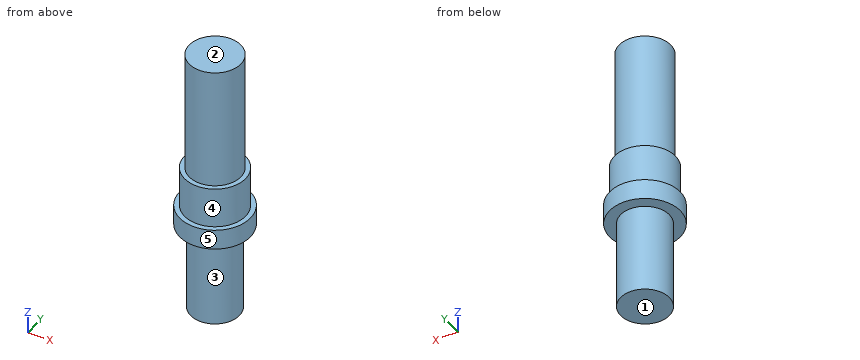
from build123d import *

# Parameters (mm, degrees)
SKETCH5_R             = 6.35
OUTSIDE_EXTRUDE_DEPTH = 30
INSIDE_START          = 2
SKETCH6_R             = 6
INSIDE_EXTRUDE_DEPTH  = 2


with BuildPart() as part:
    # Sketch3 → Initial Resolve -- Exact Length (revolve)
    with BuildSketch(Plane(origin=(0, 0, 0), x_dir=(0, 0, -1), z_dir=(1, 0, 0))):
        Polygon((9.998219577, 8.7), (14.998219577, 8.7), (14.998219577, 6), (34.998219577, 6), (34.998219577, 0), (0, 0), (-0.001780423, 0), (-0.001780423, 7.5), (9.998219577, 7.5), align=None)
    revolve(axis=Axis((0, 0, -34.998219577), (0, 0, 1)))

    # Sketch5 → Outside Extrude (add)
    with BuildSketch(Plane.XY.offset(0.001780423)):
        Circle(SKETCH5_R)
    extrude(amount=OUTSIDE_EXTRUDE_DEPTH)

    # Sketch6 → Inside Extrude (add)
    with BuildSketch(Plane(origin=(0, 0, -34.998219577), x_dir=(-1, 0, 0), z_dir=(0, 0, -1)).offset(INSIDE_START)):
        with Locations(Location((0, 0, 0), (0, 0, 90))):
            Circle(SKETCH6_R)
    extrude(amount=-INSIDE_EXTRUDE_DEPTH)


solid = part.part
Model file for the job. Use its own axes, mm. Face numbers are marked on the shaded views. A direction names the side the tool comes from. Give positions to 0.01 mm unless a question says otherwise; leave off trailing zeros. Loops run counter-clockwise (first coordinate to the right, second up) from the corner with the lowest first, then second, coordinate; pieces in that order, holes last.
1) Wall check: line 1 (Z direction, x = 4.5, y = 5.75); line 2 (Y direction, x = -5.25, z = 2); line 3 (X direction, y = -3.25, z = 26). Give the ranges that are in metal, low to high.
2) Flat gauge pins, fed straight in: pin 1 Ø10 at (y, z) = (3.5, -23) entering from -X; pin 2 Ø3 at (y, z) = (-0.5, 5.5) entering from -X; pin 3 Ø4 at (y, z) = (5, -27.5) entering from -X. Where does each tip first touch, or does it go through?
3) Saw through at A-A (x = 0). Write the cut outline in (y, z).
4) Tool access for the marked faces 4 and 5: list every direction of +Z, -Z, +X, -X, +Y, -Y with a clear straight run to the whole face (end or side of a thin tool).
5) Pull direction Z, two halves, no side cores. Call the marked faces 1, 2 and 3: +Z half, -Z half, draft (parallel to the pull), parting line (faces both ways), or undercut.
6) Saw through at C-C (z = 6). Write the cut outline in (x, y), plus the area to 3 significant figures.
7) Saw through at D-D (z = -3.5). Write the cut outline in (x, y), plus the area to 3 significant figures.
Answer block:
1. line 1: z = -15 to 0
1. line 2: y = -3.57 to 3.57
1. line 3: x = -5.46 to 5.46
2. pin 1: stops at x = -6
2. pin 2: stops at x = -6.35
2. pin 3: stops at x = -5.2
3. outline: (-8.7, -15) - (-6, -15) - (-6, -37) - (6, -37) - (6, -15) - (8.7, -15) - (8.7, -10) - (7.5, -10) - (7.5, 0) - (6.35, 0) - (6.35, 30) - (-6.35, 30) - (-6.35, 0) - (-7.5, 0) - (-7.5, -10) - (-8.7, -10) - close
4. face 4: +Z
4. face 5: +Z, -Z
5. face 1: -Z half
5. face 2: +Z half
5. face 3: draft
6. outline: circle Ø12.7 at (0, 0)
6. area: 127 mm2
7. outline: circle Ø15 at (0, 0)
7. area: 177 mm2
